Geometry check sheet. Reference: the model listing, model coordinates, mm. A direction names the side the tool comes from. Give positions to 0.01 mm unless a question says otherwise; leave off trailing zeros. Order: outer loops, then holes, each group sorted by start corner. A loop starts at its lowest first (then second) coordinate and runs counter-clockwise, first axis right, second up. Notation, with made-up numbers: M 34.25,-5 L 89.25,-5 A17 ccw 89.25,11 Z; hole C -29,-33 d5. An arc over 180 degrees is marked long. Use CSV: the item, a comma, the result in double quotes. Start each with the question number.
from build123d import *

# Parameters (mm, degrees)
SKETCH_1_W                = 60
SKETCH_1_H                = 50
EXTRUDE_1_DEPTH           = 10
HOLE_WIZARD_1_D           = 8.5
HOLE_WIZARD_1_DEPTH       = 20
HOLE_WIZARD_2_D           = 8
HOLE_WIZARD_2_CSINK_D     = 8.2
HOLE_WIZARD_2_CSINK_ANGLE = 45
SKETCH_9_R                = 2.5
EXTRUDE_3_DEPTH           = 4
HOLE_WIZARD_3_D           = 3.2
CHAMFER_1_SIZE            = 4
SKETCH_15_R               = 1.6
CUT_EXTRUDE_1_DEPTH       = 41.311288741
SKETCH_16_W               = 60
SKETCH_16_H               = 10
EXTRUDE_4_DEPTH           = 10.5
SKETCH_17_W               = 80
SKETCH_17_H               = 30
EXTRUDE_5_DEPTH           = 4
SKETCH_18_R               = 1.75
EXTRUDE_6_DEPTH           = 5


with BuildPart() as part:
    # 草图1 → 凸台-拉伸1 (new body)
    with BuildSketch(Plane.XY):
        Rectangle(SKETCH_1_W, SKETCH_1_H)
    extrude(amount=EXTRUDE_1_DEPTH)

    # 孔1
    with Locations(Plane.XY.offset(10)):
        with Locations((0, 0)):
            Hole(HOLE_WIZARD_1_D / 2, depth=HOLE_WIZARD_1_DEPTH)

    # 孔2 (through all)
    with Locations(Plane.XY.offset(10)):
        with Locations((20, 0), (-20, 0)):
            CounterSinkHole(HOLE_WIZARD_2_D / 2, HOLE_WIZARD_2_CSINK_D / 2, counter_sink_angle=HOLE_WIZARD_2_CSINK_ANGLE)

    # 草图9 → 凸台-拉伸3 (add)
    with BuildSketch(Plane.XY.offset(10)):
        with Locations(Location((0, 18.25, 0), (0, 0, 180))):
            Circle(SKETCH_9_R)
        with Locations(Location((0, -18.25, 0), (0, 0, 180))):
            Circle(SKETCH_9_R)
    extrude(amount=EXTRUDE_3_DEPTH)

    # 孔3 (through all)
    with Locations(Plane.XY.offset(14)):
        with Locations((0, 18.25), (0, -18.25)):
            Hole(HOLE_WIZARD_3_D / 2)

    # 倒角1
    chamfer_1_edges = [part.edges().sort_by_distance(p)[0] for p in [
        (30, -25, 5),
        (-30, -25, 5),
    ]]
    chamfer(chamfer_1_edges, length=CHAMFER_1_SIZE)

    # 草图15 → 切除-拉伸1 (cut, through all)
    with BuildSketch(Plane.XY.offset(10)):
        with BuildLine():
            ThreePointArc((-21.13137085, 21.13137085), (-21.13137085, 18.86862915), (-18.86862915, 18.86862915))
            Line((-18.86862915, 18.86862915), (-21.13137085, 21.13137085))
        make_face()
        with BuildLine():
            Line((-21.13137085, 21.13137085), (-18.86862915, 18.86862915))
            ThreePointArc((-18.86862915, 18.86862915), (-18.521792748, 19.387706508), (-18.4, 20))
            ThreePointArc((-18.4, 20), (-19.387706508, 21.478207252), (-21.13137085, 21.13137085))
        make_face()
        with Locations((20, 20)):
            Circle(SKETCH_15_R)
        with Locations((20, -20)):
            Circle(SKETCH_15_R)
        with Locations(Location((-20, -20, 0), (0, 0, 180))):
            Circle(SKETCH_15_R)
    extrude(amount=-CUT_EXTRUDE_1_DEPTH, mode=Mode.SUBTRACT)

    # 草图16 → 凸台-拉伸4 (add)
    with BuildSketch(Plane(origin=(0, 25, 0), x_dir=(1, 0, 0), z_dir=(0, 1, 0))):
        with Locations((0, -5)):
            Rectangle(SKETCH_16_W, SKETCH_16_H)
    extrude(amount=EXTRUDE_4_DEPTH)

    # 草图17 → 凸台-拉伸5 (add)
    with BuildSketch(Plane(origin=(0, 35.5, 0), x_dir=(1, 0, 0), z_dir=(0, 1, 0))):
        with Locations((0, -15)):
            Rectangle(SKETCH_17_W, SKETCH_17_H)
    extrude(amount=-EXTRUDE_5_DEPTH)

    # 草图18 → 凸台-拉伸6 (add)
    with BuildSketch(Plane(origin=(0, 35.5, 0), x_dir=(1, 0, 0), z_dir=(0, 1, 0))):
        with Locations(Location((32, -5, 0), (0, 0, 270))):
            Circle(SKETCH_18_R)
        with Locations(Location((-18, -5, 0), (0, 0, 270))):
            Circle(SKETCH_18_R)
    extrude(amount=EXTRUDE_6_DEPTH)


solid = part.part
(1) Draft check along Y on faces 1 (the face through (19.792, -18.414, 5.07)), 2 (the face through (-40, 34, 15)), 3 (the face through (-18, 40.5, 5)), 4 (the face through (0.33, -20.73, 11.97)). Enter one of: +Y half, -Y half, draft (parallel to the pull), parting line (faces both ways), or undercut.
(2) Sectioned sample at B-B on z = 2. Give the number of separate pieces and of enclosed holes in the cut face, then the cut area to 3 significant figures.
(3) Sectioned sample at D-D on x = 32. Record the cut outline in (y, z), then the cut area to 4 significant figures.
(4) Go/stop test with flat-tipped pins: P1, Ø5, axis at x = 7.5, z = 26, coming from the +Y side; P2, Ø8, axis at x = 27.5, y = 8, coming from the +Z side; P3, Ø17, axis at x = -8.5, y = 15.5, coming from the +Z side. Record where each tip stops, or that it passes through.
(5) Thickness scan on line 1 (Y direction, x = 0, z = 9.75); line 2 (Y direction, x = -20, z = 7); line 3 (X direction, y = -18.5, z = 12.25). Record the ranges inside material, lowest first.
(6) Access from +Z, -Z, +X, -X, +Y, -Y to the whole of each face (thin tool, end or side, straight path). Record for faces 5 (the face through (33.18, 37.97, 3.71)), 6 (the face through (-30, 5, 5)), 7 (the face through (30, 5, 5)).
(7) Sectioned sample at A-A on x = 20. Record the cut outline in (y, z).
(8) Sectioned sample at C-C on x = 0. Record the cut outline in (y, z).
Responses:
1,face 1,"undercut"
1,face 2,"draft"
1,face 3,"+Y half"
1,face 4,"undercut"
2,separate pieces,"1"
2,enclosed holes,"9"
2,area,"3,490 mm2"
3,outline,"M 31.5,0 L 35.5,0 L 35.5,3.25 L 40.5,3.25 L 40.5,6.75 L 35.5,6.75 L 35.5,30 L 31.5,30 Z"
3,area,"137.5 mm2"
4,P1,"y = 35.5"
4,P2,"z = 10"
4,P3,"z = 14"
5,line 1,"-25 to -19.85, -16.65 to -4.25, 4.25 to 16.65, 19.85 to 35.5"
5,line 2,"-25 to -21.6, -18.4 to -4, 4 to 18.4, 21.6 to 35.5"
5,line 3,"-2.49 to -1.58, 1.58 to 2.49"
6,face 5,"+Y"
6,face 6,"+Z, -Z, -X, -Y"
6,face 7,"+Z, -Z, +X, -Y"
7,outline,"M -25,0 L -21.6,0 L -21.6,10 L -25,10 Z; M -18.4,0 L -4,0 L -4,9.76 L -4.1,10 L -18.4,10 Z; M 4,0 L 18.4,0 L 18.4,10 L 4.1,10 L 4,9.76 Z; M 21.6,0 L 35.5,0 L 35.5,30 L 31.5,30 L 31.5,10 L 21.6,10 Z"
8,outline,"M -25,0 L -19.85,0 L -19.85,14 L -20.75,14 L -20.75,10 L -25,10 Z; M -16.65,0 L -4.25,0 L -4.25,10 L -15.75,10 L -15.75,14 L -16.65,14 Z; M 4.25,0 L 16.65,0 L 16.65,14 L 15.75,14 L 15.75,10 L 4.25,10 Z; M 19.85,0 L 35.5,0 L 35.5,30 L 31.5,30 L 31.5,10 L 20.75,10 L 20.75,14 L 19.85,14 Z"
